Model file for the job. Use its own axes, mm. Face numbers are marked on the shaded views. Give positions to 0.01 mm unless a question says otherwise; leave off trailing zeros. Loops run counter-clockwise (first coordinate to the right, second up) from the corner with the lowest first, then second, coordinate; pieces in that order, holes last. Notation, with made-up numbers: (-30, 82.5) -> (29, 82.5) arc R17 ccw to (29, 97.5) -> close; hole circle Ø9 at (-22, 64.5). An arc over 180 degrees is marked (long way). Use CSV: the item, a comma, the result in double quotes. Start each with the question number.
(1) Pull direction X, two halves, no side cores. Call the marked faces 1, 2 and 3: pulls with the +X half, pulls with the -X half, needs draft (parallel to the pull), parting line crosses it, or undercut.
(2) Cut at C-C on z = -37.5. Write the cut outline in (x, y).
(3) Cut at B-B on z = 0. Write the cut outline in (x, y).
(4) Cut at A-A on x = 0. Write the cut outline in (y, z), then the cut area to 4 significant figures.
(5) Cut at D-D on y = -5.25. Write the cut outline in (x, z).
(6) Drill centre lines: probe 1 along Z at (x, y) = (0, -13.7); probe 2 along Z at (x, y) = (0, -6.25); probe 3 along X at (y, z) = (-1.5, 32.5). Where is each one in solid material? Low to high.
(7) Flat gauge pins, fed straight in: pin 1 (1.5 mm diameter, centred on x = 61.5, y = -4.5, fed in from -Z); pin 2 (4 mm diameter, centred on y = -8, z = -46, fed in from +X); pin 3 (1 mm diameter, centred on x = -12, y = -7, fed in from -Z). Where does each tip first touch, or does it go through?
from build123d import *

# Parameters (mm, degrees)
F0_R     = 75.5
F0_R_2   = 20
F1_DEPTH = 10
F0_R_3   = 78
F2_DEPTH = 15


with BuildPart() as f1:
    # F0 (on Front) → F1 (new body)
    with BuildSketch(Plane.XZ):
        Circle(F0_R)
        with Locations((-36.258319, -33.303391)):
            Circle(F0_R_2, mode=Mode.SUBTRACT)
        with Locations((36.258319, -33.303391)):
            Circle(F0_R_2, mode=Mode.SUBTRACT)
        with Locations((-36.258319, 33.303391)):
            Circle(F0_R_2, mode=Mode.SUBTRACT)
        Circle(F0_R_2, mode=Mode.SUBTRACT)
        with Locations((36.258319, 33.303391)):
            Circle(F0_R_2, mode=Mode.SUBTRACT)
    extrude(amount=F1_DEPTH)

    # F0 (on Front) → F2 (join)
    with BuildSketch(Plane.XZ):
        Circle(F0_R_3)
        Circle(F0_R, mode=Mode.SUBTRACT)
    extrude(amount=F2_DEPTH)


solid = f1.part
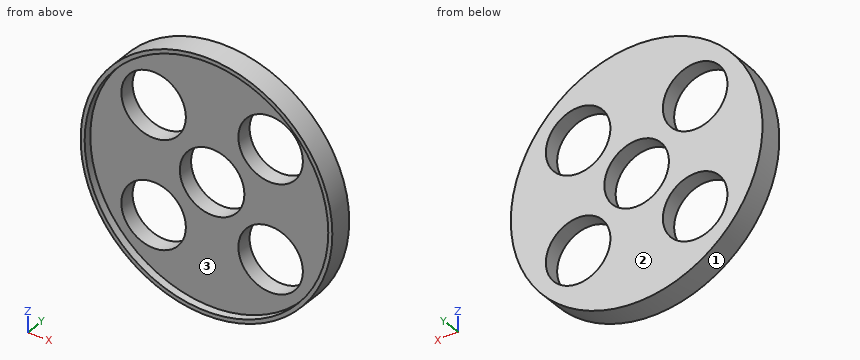
Check result:
1,face 1,"parting line crosses it"
1,face 2,"needs draft"
1,face 3,"undercut"
2,outline,"(-68.39, -15) -> (-65.53, -15) -> (-65.53, -10) -> (-55.81, -10) -> (-55.81, 0) -> (-68.39, 0) -> close; (-16.7, -10) -> (16.7, -10) -> (16.7, 0) -> (-16.7, 0) -> close; (55.81, -10) -> (65.53, -10) -> (65.53, -15) -> (68.39, -15) -> (68.39, 0) -> (55.81, 0) -> close"
3,outline,"(-78, -15) -> (-75.5, -15) -> (-75.5, -10) -> (-20, -10) -> (-20, 0) -> (-78, 0) -> close; (20, -10) -> (75.5, -10) -> (75.5, -15) -> (78, -15) -> (78, 0) -> (20, 0) -> close"
4,outline,"(-15, -78) -> (0, -78) -> (0, -20) -> (-10, -20) -> (-10, -75.5) -> (-15, -75.5) -> close; (-15, 75.5) -> (-10, 75.5) -> (-10, 20) -> (0, 20) -> (0, 78) -> (-15, 78) -> close"
4,area,"1,185 mm²"
5,outline,"circle Ø156 at (0, 0); hole circle Ø40 at (-36.26, -33.3); hole circle Ø40 at (-36.26, 33.3); hole circle Ø40 at (0, 0); hole circle Ø40 at (36.26, -33.3); hole circle Ø40 at (36.26, 33.3)"
6,probe 1,"-78 to -75.5, 75.5 to 78"
6,probe 2,"-78 to -20, 20 to 78"
6,probe 3,"-70.91 to -56.24, -16.27 to 16.27, 56.24 to 70.91"
7,pin 1,"z = -48.92"
7,pin 2,"x = 64.4"
7,pin 3,"z = -77.15"
